The model under review builds one solid part; all positions refer to its coordinate system, in mm. A direction names the side the tool comes from. Give positions to 0.01 mm unless a question says otherwise; leave off trailing zeros. Write each loop counter-clockwise with the first axis right and the second up, starting at its lowest first coordinate (ties: lowest second). Pieces come first, ordered by that corner, then holes. Notation, with made-up numbers: (-31.5, 29) -> (6.5, 29) arc R17 ccw to (6.5, 34) -> close; hole circle Ø5 at (81, -19). An arc over 180 degrees is marked (long way). Use CSV: the item, a comma, the result in double quotes.
```python
from build123d import *

# Parameters (mm, degrees)
SKIZZE2_W                            = 100
SKIZZE2_H                            = 39.364160046
AUFSATZ_LINEAR_AUSTRAGEN1_DEPTH      = 30
SCHNITT_LINEAR_AUSTRAGEN1_DEPTH      = 40
SCHNITT_LINEAR_AUSTRAGEN1_DEPTH_BACK = 40
SKIZZE10_R                           = 5
SKIZZE17_R                           = 1.4
SCHNITT_LINEAR_AUSTRAGEN2_DEPTH      = 103.710939516
SKIZZE24_R                           = 1.55
SCHNITT_LINEAR_AUSTRAGEN4_DEPTH      = 112.577493681
SKIZZE37_R                           = 0.736865544
SCHNITT_LINEAR_AUSTRAGEN9_DEPTH      = 112.577493681
SKIZZE40_R                           = 2.1
SCHNITT_LINEAR_AUSTRAGEN10_DEPTH     = 6
SKIZZE42_R                           = 0.75
SCHNITT_LINEAR_AUSTRAGEN12_DEPTH     = 10
VERRUNDUNG1_R                        = 1
SKIZZE46_R                           = 2.85
SCHNITT_LINEAR_AUSTRAGEN15_DEPTH     = 10
SCHNITT_LINEAR_START                 = -5
SCHNITT_LINEAR_AUSTRAGEN25_DEPTH     = 2.7
LINEARES_MUSTER1_COUNT               = 5
LINEARES_MUSTER1_PITCH               = 17
SPIEGELN2_COPY_1_SKETCH_R            = 2.85
SPIEGELN2_COPY_1_DEPTH               = 10
SPIEGELN2_COPY_2_SKETCH_R            = 2.85
SPIEGELN2_COPY_2_DEPTH               = 10
SPIEGELN2_COPY_3_SKETCH_R            = 2.85
SPIEGELN2_COPY_3_DEPTH               = 10
SPIEGELN2_COPY_4_SKETCH_R            = 2.85
SPIEGELN2_COPY_4_DEPTH               = 10
SPIEGELN2_START                      = -5
SPIEGELN2_COPY_5_DEPTH               = 2.7
SPIEGELN2_COPY_6_DEPTH               = 2.7
SPIEGELN2_COPY_7_DEPTH               = 2.7
SPIEGELN2_COPY_8_DEPTH               = 2.7
SCHNITT_LINEAR_START_2               = -10
SKIZZE51_R                           = 1.55
SCHNITT_LINEAR_AUSTRAGEN26_DEPTH     = 10


with BuildPart() as part:
    # Skizze2 → Aufsatz-Linear austragen1 (new body)
    with BuildSketch(Plane.XY):
        with Locations((50, 19.682080023)):
            Rectangle(SKIZZE2_W, SKIZZE2_H)
    extrude(amount=AUFSATZ_LINEAR_AUSTRAGEN1_DEPTH)

    # Skizze10 → Schnitt-Linear austragen1 (cut, two sides: drawn at the far end of the back side and taken through both)
    with BuildSketch(Plane.ZY.offset(-50).offset(-SCHNITT_LINEAR_AUSTRAGEN1_DEPTH_BACK)):
        with Locations((14.945770016, 20.027045739)):
            Circle(SKIZZE10_R)
    extrude(amount=SCHNITT_LINEAR_AUSTRAGEN1_DEPTH + SCHNITT_LINEAR_AUSTRAGEN1_DEPTH_BACK, mode=Mode.SUBTRACT)

    # Skizze17 → Schnitt-Linear austragen2 (cut, through all)
    with BuildSketch(Plane.ZY.offset(-90)):
        with Locations((14.945770016, 20.027045739)):
            Circle(SKIZZE17_R)
    schnitt_linear_austragen2 = extrude(amount=-SCHNITT_LINEAR_AUSTRAGEN2_DEPTH, mode=Mode.SUBTRACT)

    # Spiegeln1: Schnitt-Linear austragen2 across plane
    add(schnitt_linear_austragen2.mirror(Plane.ZY.offset(-50)), mode=Mode.SUBTRACT)

    # Skizze24 → Schnitt-Linear austragen4 (cut, through all)
    with BuildSketch(Plane.XY.offset(30)):
        with Locations((16, 31.364160046)):
            Circle(SKIZZE24_R)
        with Locations((33, 31.364160046)):
            Circle(SKIZZE24_R)
        with Locations((50, 31.364160046)):
            Circle(SKIZZE24_R)
        with Locations((67, 31.364160046)):
            Circle(SKIZZE24_R)
        with Locations((84, 31.364160046)):
            Circle(SKIZZE24_R)
    schnitt_linear_austragen4 = extrude(amount=-SCHNITT_LINEAR_AUSTRAGEN4_DEPTH, mode=Mode.SUBTRACT)

    # Skizze37 → Schnitt-Linear austragen9 (cut, through all)
    with BuildSketch(Plane(origin=(100, 0, 0), x_dir=(0, 0, -1), z_dir=(1, 0, 0))):
        with Locations((-18.924590299, 18.633559666)):
            Circle(SKIZZE37_R)
    extrude(amount=-SCHNITT_LINEAR_AUSTRAGEN9_DEPTH, mode=Mode.SUBTRACT)

    # Skizze40 → Schnitt-Linear austragen10 (cut)
    with BuildSketch(Plane(origin=(100, 0, 0), x_dir=(0, 0, -1), z_dir=(1, 0, 0))):
        with Locations((-18.924590299, 18.633559666)):
            Circle(SKIZZE40_R)
    extrude(amount=-SCHNITT_LINEAR_AUSTRAGEN10_DEPTH, mode=Mode.SUBTRACT)

    # Skizze42 → Schnitt-Linear austragen12 (cut)
    with BuildSketch(Plane.ZY):
        with Locations((10.86415918, 18.842582577)):
            Circle(SKIZZE42_R)
    extrude(amount=-SCHNITT_LINEAR_AUSTRAGEN12_DEPTH, mode=Mode.SUBTRACT)

    # Verrundung1
    verrundung1_edges = [part.edges().sort_by_distance(p)[0] for p in [
        (94, 18.633559666, 19.661455843),
    ]]
    fillet(verrundung1_edges, radius=VERRUNDUNG1_R)

    # Skizze46 → Schnitt-Linear austragen15 (cut)
    with BuildSketch(Plane(origin=(0, 0, 0), x_dir=(-1, 0, 0), z_dir=(0, 0, -1))):
        with Locations((-84, 31.364160046)):
            Circle(SKIZZE46_R)
    schnitt_linear_austragen15 = extrude(amount=-SCHNITT_LINEAR_AUSTRAGEN15_DEPTH, mode=Mode.SUBTRACT)

    # Skizze50 → Schnitt-Linear austragen25 (cut)
    with BuildSketch(Plane.XY.offset(30).offset(SCHNITT_LINEAR_START)):
        Polygon((81.15, 33.009608314), (81.15, 39.364160046), (86.85, 39.364160046), (86.85, 33.009608314), (86.85, 29.718711779), (84, 28.073263512), (81.15, 29.718711779), align=None)
    schnitt_linear_austragen25 = extrude(amount=-SCHNITT_LINEAR_AUSTRAGEN25_DEPTH, mode=Mode.SUBTRACT)

    # Lineares Muster1: Schnitt-Linear austragen15, Schnitt-Linear austragen25 ×5
    with Locations(*[(-i * LINEARES_MUSTER1_PITCH, 0, 0) for i in range(1, LINEARES_MUSTER1_COUNT)]):
        add(schnitt_linear_austragen15, mode=Mode.SUBTRACT)
        add(schnitt_linear_austragen25, mode=Mode.SUBTRACT)

    # Spiegeln2: Schnitt-Linear austragen15, Schnitt-Linear austragen25 across plane
    add(schnitt_linear_austragen15.mirror(Plane.ZX.offset(19.764160046)), mode=Mode.SUBTRACT)
    add(schnitt_linear_austragen25.mirror(Plane.ZX.offset(19.764160046)), mode=Mode.SUBTRACT)

    # Spiegeln2 copy 1 sketch → Spiegeln2 copy 1 (cut)
    with BuildSketch(Plane(origin=(-17, 39.528320093, 0), x_dir=(-1, 0, 0), z_dir=(0, 0, -1))):
        with Locations((-84, -31.364160046)):
            Circle(SPIEGELN2_COPY_1_SKETCH_R)
    extrude(amount=-SPIEGELN2_COPY_1_DEPTH, mode=Mode.SUBTRACT)

    # Spiegeln2 copy 2 sketch → Spiegeln2 copy 2 (cut)
    with BuildSketch(Plane(origin=(-34, 39.528320093, 0), x_dir=(-1, 0, 0), z_dir=(0, 0, -1))):
        with Locations((-84, -31.364160046)):
            Circle(SPIEGELN2_COPY_2_SKETCH_R)
    extrude(amount=-SPIEGELN2_COPY_2_DEPTH, mode=Mode.SUBTRACT)

    # Spiegeln2 copy 3 sketch → Spiegeln2 copy 3 (cut)
    with BuildSketch(Plane(origin=(-51, 39.528320093, 0), x_dir=(-1, 0, 0), z_dir=(0, 0, -1))):
        with Locations((-84, -31.364160046)):
            Circle(SPIEGELN2_COPY_3_SKETCH_R)
    extrude(amount=-SPIEGELN2_COPY_3_DEPTH, mode=Mode.SUBTRACT)

    # Spiegeln2 copy 4 sketch → Spiegeln2 copy 4 (cut)
    with BuildSketch(Plane(origin=(-68, 39.528320093, 0), x_dir=(-1, 0, 0), z_dir=(0, 0, -1))):
        with Locations((-84, -31.364160046)):
            Circle(SPIEGELN2_COPY_4_SKETCH_R)
    extrude(amount=-SPIEGELN2_COPY_4_DEPTH, mode=Mode.SUBTRACT)

    # Spiegeln2 copy 5 sketch → Spiegeln2 copy 5 (cut)
    with BuildSketch(Plane(origin=(-17, 39.528320093, 30), x_dir=(1, 0, 0), z_dir=(0, 0, 1)).offset(SPIEGELN2_START)):
        Polygon((81.15, -33.009608314), (81.15, -39.364160046), (86.85, -39.364160046), (86.85, -33.009608314), (86.85, -29.718711779), (84, -28.073263512), (81.15, -29.718711779), align=None)
    extrude(amount=-SPIEGELN2_COPY_5_DEPTH, mode=Mode.SUBTRACT)

    # Spiegeln2 copy 6 sketch → Spiegeln2 copy 6 (cut)
    with BuildSketch(Plane(origin=(-34, 39.528320093, 30), x_dir=(1, 0, 0), z_dir=(0, 0, 1)).offset(SPIEGELN2_START)):
        Polygon((81.15, -33.009608314), (81.15, -39.364160046), (86.85, -39.364160046), (86.85, -33.009608314), (86.85, -29.718711779), (84, -28.073263512), (81.15, -29.718711779), align=None)
    extrude(amount=-SPIEGELN2_COPY_6_DEPTH, mode=Mode.SUBTRACT)

    # Spiegeln2 copy 7 sketch → Spiegeln2 copy 7 (cut)
    with BuildSketch(Plane(origin=(-51, 39.528320093, 30), x_dir=(1, 0, 0), z_dir=(0, 0, 1)).offset(SPIEGELN2_START)):
        Polygon((81.15, -33.009608314), (81.15, -39.364160046), (86.85, -39.364160046), (86.85, -33.009608314), (86.85, -29.718711779), (84, -28.073263512), (81.15, -29.718711779), align=None)
    extrude(amount=-SPIEGELN2_COPY_7_DEPTH, mode=Mode.SUBTRACT)

    # Spiegeln2 copy 8 sketch → Spiegeln2 copy 8 (cut)
    with BuildSketch(Plane(origin=(-68, 39.528320093, 30), x_dir=(1, 0, 0), z_dir=(0, 0, 1)).offset(SPIEGELN2_START)):
        Polygon((81.15, -33.009608314), (81.15, -39.364160046), (86.85, -39.364160046), (86.85, -33.009608314), (86.85, -29.718711779), (84, -28.073263512), (81.15, -29.718711779), align=None)
    extrude(amount=-SPIEGELN2_COPY_8_DEPTH, mode=Mode.SUBTRACT)

    # Spiegeln3: Schnitt-Linear austragen4 across plane
    add(schnitt_linear_austragen4.mirror(Plane.ZX.offset(19.764160046)), mode=Mode.SUBTRACT)

    # Skizze51 → Schnitt-Linear austragen26 (cut)
    with BuildSketch(Plane.XY.offset(30).offset(SCHNITT_LINEAR_START_2)):
        with Locations((5, 34.364160046)):
            Circle(SKIZZE51_R)
        with Locations((95, 5)):
            Circle(SKIZZE51_R)
    extrude(amount=-SCHNITT_LINEAR_AUSTRAGEN26_DEPTH, mode=Mode.SUBTRACT)


solid = part.part
```
Q1. Machinability: for faces 4 (the flat face through (48.8, 6.9, 10)), 5 (the flat face through (64.15, 35, 24)), 6 (the flat face through (81.15, 5, 24)), which of the approach directions +Z, -Z, +X, -X, +Y, -Y give a long, thin tool a straight path to every point of the face, cutting with its end or side? Answer none if there is none.
Derived:
face 4,"-Z"
face 5,"+Y"
face 6,"none"
Q2. To check wall thickness, follow probe 1 along Y at (x, z) = (67, 28.5); probe 2 along Y at (x, z) = (50, 15); probe 3 along X at (y, z) = (19, 16.75). State the ranges of each line that lie inside material, in increasing order.
Derived:
probe 1,"y = 0 to 6.61, 9.71 to 29.81, 32.91 to 39.36"
probe 2,"y = 0 to 6.61, 9.71 to 15.03, 25.03 to 29.81, 32.91 to 39.36"
probe 3,"x = 0 to 10, 90 to 100"
Q3. Consider section A-A (x = 95). Write out the cut boundary in (y, z), then the cut area to 3 significant figures.
Derived:
outline,"(0, 0) -> (39.36, 0) -> (39.36, 30) -> (0, 30) -> close; hole (3.45, 10) -> (6.55, 10) -> (6.55, 20) -> (3.45, 20) -> close; hole circle Ø4.2 at (18.63, 18.92); hole circle Ø2.8 at (20.03, 14.95)"
area,"1,130 mm2"
Q4. The part is to be moulded in two halves that separate along Z. For faces 1 (the cylindrical face through (85.43, 30.77, 27.54)), 2 (the flat face through (14.8, 6.9, 10)), 3 (the cylindrical face through (94.93, 19.18, 13.83)), say which applies: pulls with the +Z half, pulls with the -Z half, needs draft (parallel to the pull), parting line crosses it, or undercut.
Derived:
face 1,"needs draft"
face 2,"pulls with the -Z half"
face 3,"undercut"
Q5. Insertion check: pin 1 (0.8 mm diameter, centred on x = 67.5, z = 23.5, fed in from +Y); pin 2 (3 mm diameter, centred on x = 15.5, y = 7.5, fed in from -Z). Each pin has a flat end and moves straight along its axis. Give the tip position at first contact, or say it passes through.
Derived:
pin 1,"stops at y = 28.59"
pin 2,"stops at z = 10"
Q6. Consider section C-C (z = 27.5). State how many separate pieces and enclosed holes the cut face has, then the cut area to 3 significant figures.
Derived:
separate pieces,"1"
enclosed holes,"10"
area,"3,860 mm2"
Q7. Consider section B-B (x = 5). Write out the cut boundary in (y, z), then the cut area to 3 significant figures.
Derived:
outline,"(0, 0) -> (39.36, 0) -> (39.36, 30) -> (0, 30) -> close; hole circle Ø1.47 at (18.63, 18.92); hole circle Ø1.5 at (18.84, 10.86); hole circle Ø2.8 at (20.03, 14.95); hole (32.81, 10) -> (35.91, 10) -> (35.91, 20) -> (32.81, 20) -> close"
area,"1,140 mm2"
